```python
from build123d import *

# Parameters (mm, degrees)
ESQUISSE1_R        = 3
BOSS_EXTRU_1_DEPTH = 3


with BuildPart() as part:
    # Esquisse1 → Boss.-Extru.1 (new body)
    with BuildSketch(Plane.XY):
        Polygon((-130.649820486, -22.415487094), (-119.070790786, -62.796362516), (-120.442039466, -65.27016062), (-138.268849115, -70.381916029), (-140.742647218, -69.010667349), (-154.419403971, -21.314148304), (-164.521687886, -13.701531345), (-206.306232172, -13.701531345), (-228.687205956, -7.283890383), (-246.894010665, -2.064269008), (-249.872259625, -3.248768002), (-288.323340616, 7.774587685), (-290.221637422, 10.357120157), (-324.023652204, 20.047657387), (-328.759186056, 17.422535954), (-351.248940808, -61.008559605), (-348.624077987, -65.743937486), (-292.570685007, -81.816989279), (-286.703799003, -97.823971184), (-249.693611115, -114.655437515), (-232.462472657, -132.451258614), (-227.051679806, -132.536382762), (-198.975350278, -105.350948678), (-136.615169465, -105.350948678), (-108.538839937, -132.536382762), (-103.128047086, -132.451258614), (-85.896908628, -114.655437515), (-48.88672074, -97.823971184), (-43.019834736, -81.816989279), (13.033558244, -65.743937486), (15.658421065, -61.008559605), (-6.831333687, 17.422535954), (-11.566867539, 20.047657387), (-45.368882322, 10.357120157), (-47.267179127, 7.774587685), (-85.718260118, -3.248768002), (-88.696509078, -2.064269008), (-106.903313787, -7.283890383), (-125.164825765, -12.52029468), align=None)
        with Locations((9.292284284, -60.574933915)):
            Circle(ESQUISSE1_R, mode=Mode.SUBTRACT)
        with Locations((-323.590068827, 13.68165837)):
            Circle(ESQUISSE1_R, mode=Mode.SUBTRACT)
        with Locations((-216.832585966, -16.924131519)):
            Circle(ESQUISSE1_R, mode=Mode.SUBTRACT)
        with Locations((-167.795259872, -27.605548894)):
            Circle(ESQUISSE1_R, mode=Mode.SUBTRACT)
        with Locations((-118.757933777, -16.924131519)):
            Circle(ESQUISSE1_R, mode=Mode.SUBTRACT)
        with Locations((-12.000450916, 13.68165837)):
            Circle(ESQUISSE1_R, mode=Mode.SUBTRACT)
        with Locations((-229.666591606, -126.713325795)):
            Circle(ESQUISSE1_R, mode=Mode.SUBTRACT)
        with Locations((-204.059552706, -101.880200807)):
            Circle(ESQUISSE1_R, mode=Mode.SUBTRACT)
        with Locations((-281.934339477, -93.401689518)):
            Circle(ESQUISSE1_R, mode=Mode.SUBTRACT)
        with Locations((-344.882804027, -60.574933915)):
            Circle(ESQUISSE1_R, mode=Mode.SUBTRACT)
        Polygon((-210.232188047, -30.001147656), (-224.390430785, -79.377961929), (-208.212806214, -96.161100182), (-207.491865187, -96.85509979), (-208.236606037, -97.572971364), (-229.533063287, -118.225792128), (-242.655085998, -104.673746846), (-258.969310369, -95.012679745), (-277.629290011, -88.825419148), (-272.289144354, -70.202118055), (-298.538981418, -62.6750984), (-299.849714513, -67.246167925), (-337.461409717, -56.461187875), (-321.404434006, -0.463858857), (-284.873898651, -10.938821309), (-283.564528345, -6.372504389), (-265.299260667, -11.609985616), (-264.679553884, -9.448811229), (-245.452786066, -14.960840928), (-246.072799476, -17.123084647), (-227.807531798, -22.360565873), (-228.496674065, -24.763890567), align=None, mode=Mode.SUBTRACT)
        with Locations((-105.923928137, -126.713325795)):
            Circle(ESQUISSE1_R, mode=Mode.SUBTRACT)
        with Locations((-131.530967037, -101.880200807)):
            Circle(ESQUISSE1_R, mode=Mode.SUBTRACT)
        with Locations((-53.656180266, -93.401689518)):
            Circle(ESQUISSE1_R, mode=Mode.SUBTRACT)
        Polygon((-106.057456456, -118.225792128), (-128.0696158, -96.878899722), (-111.200088958, -79.377961929), (-125.358331696, -30.001147656), (-107.093845678, -24.763890567), (-107.782987945, -22.360565873), (-89.517720268, -17.123084647), (-90.137733677, -14.960840928), (-70.910965859, -9.448811229), (-70.291259076, -11.609985616), (-52.025991399, -6.372504389), (-50.716621092, -10.938821309), (-14.186085737, -0.463858857), (1.870889973, -56.461187875), (-35.740805231, -67.246167925), (-37.051538325, -62.6750984), (-63.301375389, -70.202118055), (-57.961229733, -88.825419148), (-76.621209374, -95.012679745), (-92.935433745, -104.673746846), align=None, mode=Mode.SUBTRACT)
    extrude(amount=BOSS_EXTRU_1_DEPTH)


solid = part.part
```
Verification items for the finished model (mm, model axes). A direction names the side the tool comes from. Round coordinates to 2 decimals unless told otherwise and drop trailing zeros. Write each loop counter-clockwise with the first axis right and the second up, starting at its lowest first coordinate (ties: lowest second). Pieces come first, ordered by that corner, then holes. Notation, with made-up numbers: (19.25, 73.25) - (33.25, 73.25) arc R33 ccw to (33.25, 104.25) - close; hole circle Ø4 at (71, 8.25). An arc over 180 degrees is marked (long way). Answer as a JSON object with one key per item and string values. Group by question number.
Q1. Mould release check, pull along Y, two halves, no side actions. Record for faces 1 (the flat face through (-218.736, -107.755, 1.479)), 2 (the flat face through (4.57, -22.34, 1.48)), 3 (the flat face through (-119.8, -88.3, 1.5)), 4 (the flat face through (-170, -55, 3)): released by +Y, released by -Y, zero draft, split by the parting line, or undercut.
Q2. Thickness scan on line 1 (X direction, y = -50, z = 0.65); line 2 (X direction, y = -108, z = 0.8); line 3 (Y direction, x = -315, z = 2.45). Record the ranges inside material, lowest first.
Q3. Section check B-B, the plane z = 1.25. Give the number of separate pieces and of enclosed holes in the cut face, plus the area to 3 significant figures.
Q4. Section check C-C, the plane x = -144.5. Enter the section's corners in (y, z).
Q5. Go/stop test with flat-tipped pins: pin 1 Ø5.5 at (x, y) = (-12, 13.68) entering from -Z; pin 2 Ø9.5 at (x, y) = (-105.92, -126.71) entering from +Z; pin 3 Ø1 at (y, z) = (-13, 2.5) entering from -X; pin 4 Ø1.5 at (x, z) = (-195.5, 2) entering from +Y. Record where each tip stops, or that it passes through.
Q6. Section check A-A, the plane y = -37.5. Enter the section's corners in (x, z), plus the area to 3 significant figures.
Q7. Tool access check on faces 5 (the flat face through (-268.829, 2.186, 1.479)), 6 (the flat face through (-213.21, -119.134, 1.479)), 7 (the flat face through (-217.2, -54.3, 1.5)). Record the directions out of +Z, -Z, +X, -X, +Y, -Y that give a thin tool (end or side, any length) a straight path to the whole face; none if there is none.
Found:
{
 "1": {"face 1": "undercut", "face 2": "released by +Y", "face 3": "undercut", "face 4": "zero draft"},
 "2": {"line 1": "x = -348.09 to -335.61, -215.97 to -146.19, -122.74 to -119.62, 0.02 to 12.5", "line 2": "x = -264.33 to -239.43, -218.99 to -201.71, -133.88 to -116.6, -96.16 to -71.26", "line 3": "y = -75.39 to -62.9, -2.3 to 17.46"},
 "3": {"separate pieces": "1", "enclosed holes": "15", "area": "16,900 mm^2"},
 "4": {"outline": "(-105.35, 0) - (-55.91, 0) - (-55.91, 3) - (-105.35, 3) - close"},
 "5": {"pin 1": "passes through", "pin 2": "stops at z = 3", "pin 3": "stops at x = -337.63", "pin 4": "stops at y = -13.7"},
 "6": {"outline": "(-344.51, 0) - (-332.02, 0) - (-332.02, 3) - (-344.51, 3) - close; (-212.38, 0) - (-149.78, 0) - (-149.78, 3) - (-212.38, 3) - close; (-126.32, 0) - (-123.21, 0) - (-123.21, 3) - (-126.32, 3) - close; (-3.57, 0) - (8.92, 0) - (8.92, 3) - (-3.57, 3) - close", "area": "272 mm^2"},
 "7": {"face 5": "+Z, -Z, +Y", "face 6": "+Z, -Z, -Y", "face 7": "+Z, -Z"}
}
